Part model, mm, in its own coordinate system. A direction names the side the tool comes from. Round coordinates to 2 decimals unless told otherwise and drop trailing zeros. Return JSON: item names as keys, results as strings. Group by question number.
Item 1: Two-plate mould, pull along X, no slides. Class faces 4 (the face through (44, 2, 38.227)), 5 (the face through (43, 2, -11.303)), 6 (the face through (-63.5, 2, 3)): released by +X, released by -X, zero draft, split by the parting line, or undercut.
Item 2: Saw through at A-A on y = 1.45. State how many separate pieces and enclosed holes the cut face has, and give its area (3 significant figures).
Item 3: Probe probe 1 along Z at (x, y) = (44, 1.8) (3 decimals); probe 2 along Z at (x, y) = (-2.5, 1.3) (3 decimals); probe 3 along X at (y, z) = (0.95, -18.5). List the from-to ranges inside material, lowest first.
Item 4: Drop flat-ended pins along their axis: pin 1 (1.6 mm diameter, centred on x = 11.5, y = 2, fed in from +Z); pin 2 (1.6 mm diameter, centred on y = 2, z = 0, fed in from +X). Give the stop position or say it passes through.
Item 5: Tool access for faces 1 (the face through (56.896, 2, 22)), 2 (the face through (41.402, 2, 35)), 3 (the face through (-17.653, 2, 0)): list every direction of +Z, -Z, +X, -X, +Y, -Y with a clear straight run to the whole face (end or side of a thin tool).
```python
from build123d import *

# Parameters (mm, degrees)
SKETCH1_W           = 127
SKETCH1_H           = 107.95
BOSS_EXTRUDE1_DEPTH = 3.175
SKETCH2_W           = 6.604
SKETCH2_H           = 6.604
CUT_EXTRUDE1_DEPTH  = 84.400427157
SKETCH3_W           = 6.477
SKETCH3_H           = 3.302
SKETCH3_W_2         = 3.302
SKETCH3_H_2         = 3.429
SKETCH3_W_3         = 5.334
SKETCH3_W_4         = 38.1
SKETCH3_H_3         = 12.7
CUT_EXTRUDE2_DEPTH  = 84.400427157


with BuildPart() as part:
    # Sketch1 → Boss-Extrude1 (new body)
    with BuildSketch(Plane(origin=(0, 0, 0), x_dir=(1, 0, 0), z_dir=(0, 1, 0))):
        Rectangle(SKETCH1_W, SKETCH1_H)
    extrude(amount=BOSS_EXTRUDE1_DEPTH)

    # Sketch2 → Cut-Extrude1 (cut, through all)
    with BuildSketch(Plane.XZ):
        with Locations((60.198, 22.225)):
            Rectangle(SKETCH2_W, SKETCH2_H)
        Polygon((63.5, 38.227), (63.5, 31.623), (56.896, 31.623), (47.371, 31.623), (47.371, 38.227), (41.402, 38.227), (41.402, 31.623), (34.798, 31.623), (34.798, 38.227), (28.702, 38.227), (28.702, 31.623), (22.098, 31.623), (22.098, 38.227), (16.002, 38.227), (16.002, 31.623), (9.398, 31.623), (9.398, 38.227), (3.302, 38.227), (3.302, 31.623), (-3.302, 31.623), (-3.302, 38.227), (-9.398, 38.227), (-9.398, 31.623), (-16.002, 31.623), (-16.002, 38.227), (-22.098, 38.227), (-22.098, 31.623), (-28.702, 31.623), (-28.702, 38.227), (-34.798, 38.227), (-34.798, 31.623), (-41.402, 31.623), (-41.402, 38.227), (-47.371, 38.227), (-47.371, 31.623), (-56.896, 31.623), (-63.5, 31.623), (-63.5, 38.227), (-63.5, 53.975), (63.5, 53.975), align=None)
        with Locations((60.198, 9.525)):
            Rectangle(SKETCH2_W, SKETCH2_H)
        with Locations((60.198, -3.175)):
            Rectangle(SKETCH2_W, SKETCH2_H)
        with Locations((60.198, -15.875)):
            Rectangle(SKETCH2_W, SKETCH2_H)
        with Locations((60.198, -28.575)):
            Rectangle(SKETCH2_W, SKETCH2_H)
        with Locations((60.198, -41.275)):
            Rectangle(SKETCH2_W, SKETCH2_H)
        with Locations((60.198, -53.975)):
            Rectangle(SKETCH2_W, SKETCH2_H)
        with Locations((-60.198, -53.975)):
            Rectangle(SKETCH2_W, SKETCH2_H)
        with Locations((-60.198, -41.275)):
            Rectangle(SKETCH2_W, SKETCH2_H)
        with Locations((-60.198, -28.575)):
            Rectangle(SKETCH2_W, SKETCH2_H)
        with Locations((-60.198, -15.875)):
            Rectangle(SKETCH2_W, SKETCH2_H)
        with Locations((-60.198, -3.175)):
            Rectangle(SKETCH2_W, SKETCH2_H)
        with Locations((-60.198, 9.525)):
            Rectangle(SKETCH2_W, SKETCH2_H)
        with Locations((-60.198, 22.225)):
            Rectangle(SKETCH2_W, SKETCH2_H)
    extrude(amount=-CUT_EXTRUDE1_DEPTH, mode=Mode.SUBTRACT)

    # Sketch3 → Cut-Extrude2 (cut, through all)
    with BuildSketch(Plane(origin=(0, 0, 0), x_dir=(1, 0, 0), z_dir=(0, 1, 0))):
        Polygon((44.45, 24.13), (41.2115, 24.13), (41.148, 20.828), (41.148, 17.78), (44.45, 17.78), align=None)
        with Locations((41.2115, 0.381)):
            Rectangle(SKETCH3_W, SKETCH3_H)
        with Locations((42.799, 6.6675)):
            Rectangle(SKETCH3_W_2, SKETCH3_H_2)
        with Locations((42.799, 13.0175)):
            Rectangle(SKETCH3_W_2, SKETCH3_H_2)
        with Locations((30.48, 0.381)):
            Rectangle(SKETCH3_W_3, SKETCH3_H)
        with Locations((20.32, 0.381)):
            Rectangle(SKETCH3_W_3, SKETCH3_H)
        with Locations((10.16, 0.381)):
            Rectangle(SKETCH3_W_3, SKETCH3_H)
        with Locations((0, 0.381)):
            Rectangle(SKETCH3_W_3, SKETCH3_H)
        with Locations((-10.16, 0.381)):
            Rectangle(SKETCH3_W_3, SKETCH3_H)
        with Locations((-20.32, 0.381)):
            Rectangle(SKETCH3_W_3, SKETCH3_H)
        with Locations((-42.799, 13.0175)):
            Rectangle(SKETCH3_W_2, SKETCH3_H_2)
        Polygon((-44.45, 24.13), (-44.45, 17.78), (-41.148, 17.78), (-41.148, 20.828), (-41.2115, 24.13), align=None)
        with Locations((-42.799, 6.6675)):
            Rectangle(SKETCH3_W_2, SKETCH3_H_2)
        with Locations((-30.48, 0.381)):
            Rectangle(SKETCH3_W_3, SKETCH3_H)
        with Locations((-41.2115, 0.381)):
            Rectangle(SKETCH3_W, SKETCH3_H)
        with Locations((0.358722149, 11.43)):
            Rectangle(SKETCH3_W_4, SKETCH3_H_3)
    extrude(amount=CUT_EXTRUDE2_DEPTH, mode=Mode.SUBTRACT)


solid = part.part
```
Filled in:
{
 "1": {"face 4": "zero draft", "face 5": "undercut", "face 6": "released by -X"},
 "2": {"separate pieces": "1", "enclosed holes": "16", "area": "9,890 mm^2"},
 "3": {"probe 1": "z = -53.975 to -24.13, -17.78 to -14.732, -11.303 to -8.382, -4.953 to -2.032, 1.27 to 38.227", "probe 2": "z = -53.975 to -17.78, -5.08 to -2.032, 1.27 to 31.623", "probe 3": "x = -56.9 to -44.45, -41.15 to 41.15, 44.45 to 56.9"},
 "4": {"pin 1": "stops at z = 31.62", "pin 2": "stops at x = 63.5"},
 "5": {"face 1": "+X, +Y, -Y", "face 2": "+Z, +Y, -Y", "face 3": "+Y, -Y"}
}
